Geometry: final body of the model. Coordinates: model frame, mm. Face numbers are marked on the shaded views. A direction names the side the tool comes from. Coordinates: 2 decimals unless noted, no trailing zeros. Order: outer loops, then holes, each group sorted by start corner. A loop starts at its lowest first (then second) coordinate and runs counter-clockwise, first axis right, second up. Notation, with made-up numbers: M 75.25,37 L 112.25,37 A23 ccw 112.25,63 Z; hole C 40,64.5 d10. An arc over 180 degrees is marked long. One line per question, with ' | ' between items.
from build123d import *

# Parameters (mm, degrees)
F1_DEPTH = 100
F4_D     = 15


with BuildPart() as f1:
    # F0 (on Front) → F1 (new body)
    with BuildSketch(Plane.XZ):
        Polygon((29.8991873538, 23.8793696377), (29.8991873538, 18.1159283534), (33.8991873538, 18.1159283534), (33.8991873538, 26.1159283534), (33.8991873538, 30.1159283534), (-5.1008126462, 30.1159283534), (-5.1008126462, 26.1159283534), (7.3991873538, 26.1159283534), (7.3991873538, 1.1159283534), (11.3991873538, 1.1159283534), (11.3991873538, 23.8793696377), align=None)
    extrude(amount=F1_DEPTH)


with BuildPart() as f1_1:
    # F2: moved
    add(f1.part.moved(Location((0, 46.4, -0.6))))

    # F4 (through all)
    with Locations(Plane(origin=(0, 0, 0), x_dir=(0, 1, 0), z_dir=(-1, 0, 0))):
        with Locations((35.2738084853, -9.32151151), (15.8158723235, -9.44767434), (-3.6420638382, -9.57383717), (-23.1, -9.7), (-42.5579361618, -9.82616283)):
            Hole(F4_D / 2)


solid = f1_1.part
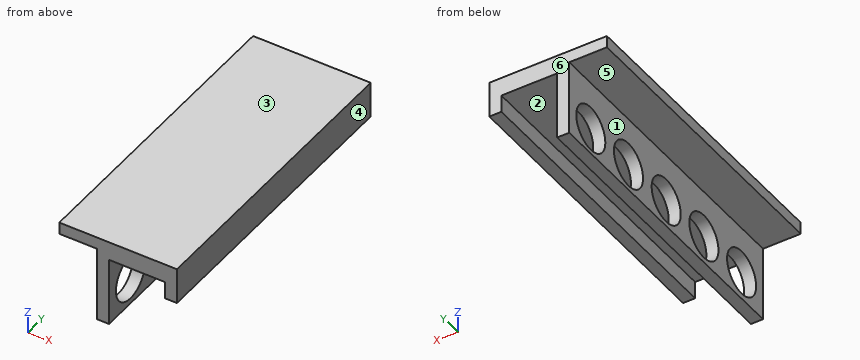
1. Section D-D, the plane z = 7. Output: boundary loops of the cut face in (x, y), and give its area (3 significant figures).
Response values:
outline: M 7.4,-53.6 L 11.4,-53.6 L 11.4,-49.51 L 7.4,-49.51 Z; M 7.4,-35.61 L 11.4,-35.61 L 11.4,-30.1 L 7.4,-30.1 Z; M 7.4,-16.1 L 11.4,-16.1 L 11.4,-10.69 L 7.4,-10.69 Z; M 7.4,3.4 L 11.4,3.4 L 11.4,8.73 L 7.4,8.73 Z; M 7.4,22.91 L 11.4,22.91 L 11.4,28.14 L 7.4,28.14 Z; M 7.4,42.41 L 11.4,42.41 L 11.4,46.4 L 7.4,46.4 Z | area: 118 mm^2
2. Pin query (flat end, axial travel): P1, Ø14, axis at x = -1.5, y = -3, coming from the -Z side; P2, Ø1.2, axis at x = 33, y = -6, coming from the -Z side; P3, Ø1.7, axis at y = 12, z = 19.5, coming from the -X side. Return the tip coordinate at first contact, or that it passes through.
Response values:
P1: stops at z = 25.52 | P2: stops at z = 17.52 | P3: stops at x = 7.4
3. Section A-A, the plane y = -23.1. Output: boundary loops of the cut face in (x, z).
Response values:
outline: M -5.1,25.52 L 7.4,25.52 L 7.4,17.2 L 11.4,17.2 L 11.4,23.28 L 29.9,23.28 L 29.9,17.52 L 33.9,17.52 L 33.9,29.52 L -5.1,29.52 Z; M 7.4,0.52 L 11.4,0.52 L 11.4,2.2 L 7.4,2.2 Z
4. Access query for the marked faces 5 and 6. Directions: +Z, -Z, +X, -X, +Y, -Y. A direction counts if a zero-diameter tool reaches every point of the face in a straight line with its end or side. Return the directions, or none.
Response values:
face 5: -Z, -X, +Y, -Y | face 6: +Z, -Z, +X, -X, +Y
5. Section B-B, the plane z = 19.5. Output: boundary loops of the cut face in (x, y), and give its area (3 significant figures).
Response values:
outline: M 7.4,-53.6 L 11.4,-53.6 L 11.4,46.4 L 7.4,46.4 Z; M 29.9,-53.6 L 33.9,-53.6 L 33.9,46.4 L 29.9,46.4 Z | area: 800 mm^2
6. Material intervals for line 1 (X direction, y = -5, z = 20); line 2 (Z direction, x = 9, y = -23); line 3 (Y direction, x = 11, z = 3.75), sorted ascending. Write a range as [from, to].
Response values:
line 1: x = [7.4, 11.4], [29.9, 33.9] | line 2: z = [0.52, 2.2], [17.2, 29.52] | line 3: y = [-53.6, -46.95], [-38.16, -27.67], [-18.53, -8.37], [1.08, 10.94], [20.69, 30.25], [40.29, 46.4]
7. Section C-C, the plane x = 9. Output: boundary loops of the cut face in (y, z), and give its area (3 significant figures).
Response values:
outline: M -53.6,0.52 L 46.4,0.52 L 46.4,29.52 L -53.6,29.52 Z; hole C -42.56,9.83 d15; hole C -23.1,9.7 d15; hole C -3.64,9.57 d15; hole C 15.82,9.45 d15; hole C 35.27,9.32 d15 | area: 2,020 mm^2
8. Draft query along X for the marked faces 1, 2, 3 and 4. Return one class per face: pulls with the +X half, pulls with the -X half, needs draft (parallel to the pull), parting line crosses it, or undercut.
Response values:
face 1: pulls with the -X half | face 2: undercut | face 3: needs draft | face 4: pulls with the +X half
